```python
from build123d import *

# Parameters (mm, degrees)
SKETCH2_W                = 254
SKETCH2_H                = 304.8
BOSS_EXTRUDE1_DEPTH      = 6.35
M4_CLEARANCE_HOLE1_D     = 4.8
M4_CLEARANCE_HOLE1_DEPTH = 6.35
SKETCH6_W                = 254
SKETCH6_H                = 6.35
BOSS_EXTRUDE2_DEPTH      = 101.6
CHAMFER1_SIZE            = 25.4
SKETCH7_W                = 66.675
SKETCH7_H                = 76.2
CUT_EXTRUDE1_DEPTH       = 7.35
CHAMFER2_SIZE            = 6.35
M5_CLEARANCE_HOLE1_D     = 5.5


with BuildPart() as part:
    # Sketch2 → Boss-Extrude1 (new body)
    with BuildSketch(Plane(origin=(0, 0, 0), x_dir=(1, 0, 0), z_dir=(0, 1, 0))):
        Rectangle(SKETCH2_W, SKETCH2_H)
    extrude(amount=BOSS_EXTRUDE1_DEPTH)

    # M4 Clearance Hole1
    with Locations(Plane(origin=(0, 6.35, 0), x_dir=(1, 0, 0), z_dir=(0, 1, 0))):
        with Locations((78.5, -111), (48.5, -111), (48.5, -143), (78.5, -143), (-48.5, -111), (-48.5, -143), (-78.5, -111), (-78.5, -143), (78.5, 143), (78.5, 111), (48.5, 143), (48.5, 111), (-48.5, 143), (-48.5, 111), (-78.5, 143), (-78.5, 111)):
            Hole(M4_CLEARANCE_HOLE1_D / 2, depth=M4_CLEARANCE_HOLE1_DEPTH)

    # Sketch6 → Boss-Extrude2 (add)
    with BuildSketch(Plane(origin=(0, 0, -152.4), x_dir=(-1, 0, 0), z_dir=(0, 0, -1))):
        with Locations((0, 3.175)):
            Rectangle(SKETCH6_W, SKETCH6_H)
    extrude(amount=BOSS_EXTRUDE2_DEPTH)

    # Chamfer1
    chamfer1_edges = [part.edges().sort_by_distance(p)[0] for p in [
        (127, 3.175, -254),
        (-127, 3.175, -254),
    ]]
    chamfer(chamfer1_edges, length=CHAMFER1_SIZE)

    # Sketch7 → Cut-Extrude1 (cut, through all)
    with BuildSketch(Plane(origin=(0, 6.35, 0), x_dir=(1, 0, 0), z_dir=(0, 1, 0))):
        with Locations((0, 215.9)):
            Rectangle(SKETCH7_W, SKETCH7_H)
    extrude(amount=-CUT_EXTRUDE1_DEPTH, mode=Mode.SUBTRACT)

    # Chamfer2
    chamfer2_edges = [part.edges().sort_by_distance(p)[0] for p in [
        (33.3375, 3.175, -254),
        (33.3375, 3.175, -177.8),
        (-33.3375, 3.175, -177.8),
        (-33.3375, 3.175, -254),
    ]]
    chamfer(chamfer2_edges, length=CHAMFER2_SIZE)

    # M5 Clearance Hole1 (through all)
    with Locations(Plane(origin=(0, 6.35, 0), x_dir=(1, 0, 0), z_dir=(0, 1, 0))):
        with Locations((-8, -20.000000026), (-8, 19.999999974), (-32, 19.999999974), (-32, -20.000000026)):
            Hole(M5_CLEARANCE_HOLE1_D / 2)


solid = part.part
```
Geometry: final body of the model. Coordinates: model frame, mm. Coordinates: 2 decimals unless noted, no trailing zeros. Write each question's results on one line, items separated by ' | '. Start each with the question number.
1) Cut plane A-A, the plane y = 2. State how many separate pieces and enclosed holes the cut face has, and give its area (3 significant figures).
2) Material intervals for line 1 along Z through (x, y) = (48.5, 3.5); line 2 along X through (y, z) = (2.5, 111); line 3 along X through (y, z) = (3.25, -185.5), sorted ascending.
3) First-contact query: pin 1 (4.5 mm diameter, centred on x = -48.5, z = -111, fed in from +Y); pin 2 (3 mm diameter, centred on x = -10, y = 3.5, fed in from -Z). Flat tips, straight axial feed; report the tip coordinate or a pass-through.
Checks:
1) separate pieces: 1 | enclosed holes: 20 | area: 97,100 mm^2
2) line 1: -254 to -145.4, -140.6 to -113.4, -108.6 to 108.6, 113.4 to 140.6, 145.4 to 152.4 | line 2: -127 to -80.9, -76.1 to -50.9, -46.1 to 46.1, 50.9 to 76.1, 80.9 to 127 | line 3: -127 to -33.34, 33.34 to 127
3) pin 1: through | pin 2: z = -177.8
